Check sheet for the modelled part. Datum: model origin and axes. Units: mm. Round coordinates to 2 decimals unless told otherwise and drop trailing zeros. Order: outer loops, then holes, each group sorted by start corner. A loop starts at its lowest first (then second) coordinate and runs counter-clockwise, first axis right, second up. Notation, with made-up numbers: (-4, 30.25) -> (17, 30.25) arc R8 ccw to (17, 43.25) -> close; hole circle Ø10 at (34, -21.75). An arc over 180 degrees is marked (long way). Use CSV: the item, a comma, the result in double quotes.
```python
from build123d import *

# Parameters (mm, degrees)
F1_DEPTH = 20
F3_D     = 39
F4_SIZE  = 3
F5_R     = 19.5
F5_R_2   = 17
F6_DEPTH = 5


with BuildPart() as f1:
    # F0 (on Front) → F1 (new body)
    with BuildSketch(Plane.XZ):
        Polygon((14.35727, -25.044004), (28.867379, -0.088241), (14.510108, 24.955763), (-14.35727, 25.044004), (-28.867379, 0.088241), (-14.510108, -24.955763), align=None)
    extrude(amount=F1_DEPTH)

    # F3 (through all)
    with Locations(Plane.XZ.offset(20)):
        with Locations((0, 0)):
            Hole(F3_D / 2)

    # F4
    f4_edges = [f1.edges().sort_by_distance(p)[0] for p in [
        (-21.612324, -20, 12.566122),
        (0.076419, -20, 24.999883),
        (21.688743, -20, 12.433761),
        (21.612324, -20, -12.566122),
        (-0.076419, -20, -24.999883),
        (-21.688743, -20, -12.433761),
        (21.688743, 0, 12.433761),
        (21.612324, 0, -12.566122),
        (-0.076419, 0, -24.999883),
        (-21.688743, 0, -12.433761),
        (-21.612324, 0, 12.566122),
        (0.076419, 0, 24.999883),
    ]]
    chamfer(f4_edges, length=F4_SIZE)

    # F5 (on face) → F6 (join)
    with BuildSketch(Plane.XZ.offset(20)):
        Circle(F5_R)
        Circle(F5_R_2, mode=Mode.SUBTRACT)
    extrude(amount=-F6_DEPTH)


solid = f1.part
```
Q1. Mould release check, pull along X, two halves, no side actions. Record for faces 1 (the face through (2.539, -7.395, 19.334)), 2 (the face through (20.196, -1.479, -11.976)), 3 (the face through (-20.23, -1.52, 12)): pulls with the +X half, pulls with the -X half, needs draft (parallel to the pull), parting line crosses it, or undercut.
Result sheet:
face 1,"undercut"
face 2,"pulls with the +X half"
face 3,"pulls with the -X half"
Q2. Go/stop test with flat-tipped pins: pin 1 (1 mm diameter, centred on y = -6.5, z = 13.5, fed in from -X); pin 2 (1 mm diameter, centred on x = -22, y = -3, fed in from +Z); pin 3 (3 mm diameter, centred on x = 21, z = 16, fed in from -Y). Record where each tip stops, or that it passes through.
Result sheet:
pin 1,"stops at x = -21.36"
pin 2,"stops at z = 12.76"
pin 3,"stops at y = -17.32"
Q3. Sectioned sample at A-A, the plane z = 12.5. Enter the section's corners in (x, y), then the cut area to 3 significant figures.
Result sheet:
outline,"(-21.65, -17) -> (-18.18, -20) -> (-11.52, -20) -> (-11.52, -15) -> (-14.97, -15) -> (-14.97, 0) -> (-18.18, 0) -> (-21.65, -3) -> close; (11.52, -20) -> (18.19, -20) -> (21.65, -17) -> (21.65, -3) -> (18.19, 0) -> (14.97, 0) -> (14.97, -15) -> (11.52, -15) -> close"
area,"281 mm^2"
Q4. Sectioned sample at D-D, the plane y = -18.5. Enter the section's corners in (x, z).
Result sheet:
outline,"(-27.14, 0.08) -> (-13.64, -23.46) -> (13.5, -23.54) -> (27.14, -0.08) -> (13.64, 23.46) -> (-13.5, 23.54) -> close; hole circle Ø34 at (0, 0)"
Q5. Scan lines: L1, parallel to Z at x = 0, y = -17.05; L2, parallel to X at y = -1.75, z = 0.5; L3, parallel to Z at x = -4, y = -15.75. Record each from-to range of solid material in increasing order.
Result sheet:
L1,"z = -24.95 to -17, 17 to 24.95"
L2,"x = -27.18 to -19.49, 19.49 to 27.09"
L3,"z = -24.99 to -16.52, 16.52 to 25.01"
Q6. Sectioned sample at C-C, the plane y = -2.25. Enter the section's corners in (x, z), then the cut area to 3 significant figures.
Result sheet:
outline,"(-28, 0.09) -> (-14.07, -24.21) -> (13.93, -24.29) -> (28, -0.09) -> (14.07, 24.21) -> (-13.93, 24.29) -> close; hole circle Ø39 at (0, 0)"
area,"843 mm^2"
Q7. Sectioned sample at B-B, the plane x = 3. Enter the section's corners in (y, z), then the cut area to 3 significant figures.
Result sheet:
outline,"(-20, -22.01) -> (-17, -25.01) -> (-3, -25.01) -> (0, -22.01) -> (0, -19.27) -> (-15, -19.27) -> (-15, -16.73) -> (-20, -16.73) -> close; (-20, 16.73) -> (-15, 16.73) -> (-15, 19.27) -> (0, 19.27) -> (0, 21.99) -> (-3, 24.99) -> (-17, 24.99) -> (-20, 21.99) -> close"
area,"237 mm^2"
